The model under review builds one solid part; all positions refer to its coordinate system, in mm. Give positions to 0.01 mm unless a question says otherwise; leave off trailing zeros. Loops run counter-clockwise (first coordinate to the right, second up) from the corner with the lowest first, then second, coordinate; pieces in that order, holes last. Notation, with made-up numbers: (-29.5, 60.25) - (12.5, 60.25) arc R28 ccw to (12.5, 91.25) - close; hole circle Ø5 at (1, 12.25). An arc over 180 degrees is marked (long way). Return JSON: item names as keys, results as strings. Group by question number.
```python
from build123d import *

# Parameters (mm, degrees)
F0_W      = 72
F0_H      = 144
F1_DEPTH  = 6
F2_R      = 8
F3_R      = 5.8
F3_R_2    = 2
F4_DEPTH  = 25
F5_W      = 25
F5_H      = 3
F6_DEPTH  = 25
F7_W      = 8.5
F7_H      = 2.6
F8_DEPTH  = 25
F9_R      = 2
F9_W      = 10
F9_H      = 2.5
F10_DEPTH = 25
F12_DEPTH = 25
F14_DEPTH = 1.5
F16_DEPTH = 1
F17_SIZE  = 0.75


with BuildPart() as f1:
    # F0 (on Top) → F1 (new body)
    with BuildSketch(Plane.XY):
        Rectangle(F0_W, F0_H)
    extrude(amount=F1_DEPTH)

    # F2
    f2_edges = [f1.edges().sort_by_distance(p)[0] for p in [
        (-36, 72, 3),
        (36, 72, 3),
        (36, -72, 3),
        (-36, -72, 3),
    ]]
    fillet(f2_edges, radius=F2_R)

    # F3 (on Top) → F4 (cut)
    with BuildSketch(Plane.XY):
        with Locations((0, 47)):
            Circle(F3_R)
        with Locations((9.6, 47)):
            Circle(F3_R_2)
    extrude(amount=-F4_DEPTH, mode=Mode.SUBTRACT)

    # F5 (on face) → F6 (cut)
    with BuildSketch(Plane.YZ.offset(36)):
        with Locations((23.8, 2.5)):
            Rectangle(F5_W, F5_H)
    extrude(amount=-F6_DEPTH, mode=Mode.SUBTRACT)

    # F7 (on face) → F8 (cut)
    with BuildSketch(Plane.XZ.offset(72)):
        with Locations((15.25, 2.2)):
            Rectangle(F7_W, F7_H)
    extrude(amount=-F8_DEPTH, mode=Mode.SUBTRACT)

    # F9 (on face) → F10 (cut)
    with BuildSketch(Plane(origin=(0, 72, 0), x_dir=(-1, 0, 0), z_dir=(0, 1, 0))):
        with Locations((-14.83, 2.5)):
            Circle(F9_R)
        with Locations((21, 2.75)):
            Rectangle(F9_W, F9_H)
    extrude(amount=-F10_DEPTH, mode=Mode.SUBTRACT)

    # F11 (on face) → F12 (cut)
    with BuildSketch(Plane.XY.offset(6)):
        with BuildLine():
            Line((28, 70), (-28, 70))
            ThreePointArc((-28, 70), (-32.2426406871, 68.2426406871), (-34, 64))
            Line((-34, 64), (-34, -64))
            ThreePointArc((-34, -64), (-32.2426406871, -68.2426406871), (-28, -70))
            Line((-28, -70), (28, -70))
            ThreePointArc((28, -70), (32.2426406871, -68.2426406871), (34, -64))
            Line((34, -64), (34, 64))
            ThreePointArc((34, 64), (32.2426406871, 68.2426406871), (28, 70))
        make_face()
    extrude(amount=-F12_DEPTH, mode=Mode.SUBTRACT)

    # F13 (on face) → F14 (join)
    with BuildSketch(Plane.XY.offset(6)):
        with BuildLine():
            Line((28, 72), (-28, 72))
            ThreePointArc((-28, 72), (-33.6568542495, 69.6568542495), (-36, 64))
            Line((-36, 64), (-36, -64))
            ThreePointArc((-36, -64), (-33.6568542495, -69.6568542495), (-28, -72))
            Line((-28, -72), (28, -72))
            ThreePointArc((28, -72), (33.6568542495, -69.6568542495), (36, -64))
            Line((36, -64), (36, 64))
            ThreePointArc((36, 64), (33.6568542495, 69.6568542495), (28, 72))
        make_face()
        with BuildLine():
            ThreePointArc((-28, -68.5), (-31.1819805153, -67.1819805153), (-32.5, -64))
            Line((-32.5, -64), (-32.5, 64))
            ThreePointArc((-32.5, 64), (-31.1819805153, 67.1819805153), (-28, 68.5))
            Line((-28, 68.5), (28, 68.5))
            ThreePointArc((28, 68.5), (31.1819805153, 67.1819805153), (32.5, 64))
            Line((32.5, 64), (32.5, -64))
            ThreePointArc((32.5, -64), (31.1819805153, -67.1819805153), (28, -68.5))
            Line((28, -68.5), (-28, -68.5))
        make_face(mode=Mode.SUBTRACT)
    extrude(amount=F14_DEPTH)

    # F15 (on face) → F16 (join)
    with BuildSketch(Plane(origin=(0, 0, 0), x_dir=(1, 0, 0), z_dir=(0, 0, -1))):
        with BuildLine():
            Line((-28, -72), (28, -72))
            ThreePointArc((28, -72), (33.6568542495, -69.6568542495), (36, -64))
            Line((36, -64), (36, 64))
            ThreePointArc((36, 64), (33.6568542495, 69.6568542495), (28, 72))
            Line((28, 72), (-28, 72))
            ThreePointArc((-28, 72), (-33.6568542495, 69.6568542495), (-36, 64))
            Line((-36, 64), (-36, -64))
            ThreePointArc((-36, -64), (-33.6568542495, -69.6568542495), (-28, -72))
        make_face()
        with BuildLine():
            ThreePointArc((28, 70), (32.2426406871, 68.2426406871), (34, 64))
            Line((34, 64), (34, -64))
            ThreePointArc((34, -64), (32.2426406871, -68.2426406871), (28, -70))
            Line((28, -70), (-28, -70))
            ThreePointArc((-28, -70), (-32.2426406871, -68.2426406871), (-34, -64))
            Line((-34, -64), (-34, 64))
            ThreePointArc((-34, 64), (-32.2426406871, 68.2426406871), (-28, 70))
            Line((-28, 70), (28, 70))
        make_face(mode=Mode.SUBTRACT)
        with BuildLine():
            Line((34, -64), (34, 64))
            ThreePointArc((34, 64), (32.2426406871, 68.2426406871), (28, 70))
            Line((28, 70), (-28, 70))
            ThreePointArc((-28, 70), (-32.2426406871, 68.2426406871), (-34, 64))
            Line((-34, 64), (-34, -64))
            ThreePointArc((-34, -64), (-32.2426406871, -68.2426406871), (-28, -70))
            Line((-28, -70), (28, -70))
            ThreePointArc((28, -70), (32.2426406871, -68.2426406871), (34, -64))
        make_face()
        with BuildLine():
            ThreePointArc((-32, 64), (-30.8284271247, 66.8284271247), (-28, 68))
            Line((-28, 68), (28, 68))
            ThreePointArc((28, 68), (30.8284271247, 66.8284271247), (32, 64))
            Line((32, 64), (32, -64))
            ThreePointArc((32, -64), (30.8284271247, -66.8284271247), (28, -68))
            Line((28, -68), (-28, -68))
            ThreePointArc((-28, -68), (-30.8284271247, -66.8284271247), (-32, -64))
            Line((-32, -64), (-32, 64))
        make_face(mode=Mode.SUBTRACT)
    extrude(amount=F16_DEPTH)

    # F17
    f17_edges = [f1.edges().sort_by_distance(p)[0] for p in [
        (30.828427, -66.828427, 0),
        (31.181981, -67.181981, 6),
    ]]
    chamfer(f17_edges, length=F17_SIZE)


solid = f1.part
```
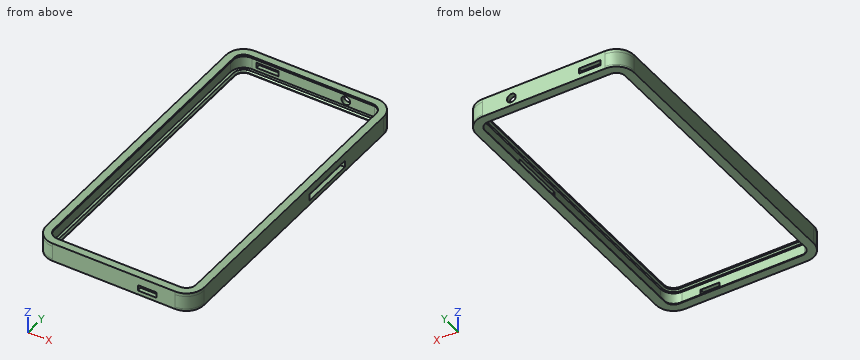
1) To check wall thickness, follow line 1 (X direction, y = -2, z = 7.25); line 2 (Y direction, x = 18.5, z = 5); line 3 (Y direction, x = -6.5, z = -0.25). State the ranges of each line that lie inside material, in increasing order.
2) For pin 1 Ø2 at (y, z) = (71, 3) entering from -X; pin 2 Ø1 at (y, z) = (19.5, 3) entering from +X; pin 3 Ø0.6 at (x, z) = (34.5, 2.5) entering from -Y, all flat-tipped, find the tip position at first contact; note any pin that passes through.
3) We need section A-A, the plane x = -2.5. Write out the cut boundary in (y, z), plus the area to 3 significant figures.
4) We need section C-C, the plane x = 14.83. Write out the cut boundary in (y, z).
5) We need section B-B, the plane y = 7. Write out the cut boundary in (x, z), plus the area to 3 significant figures.
6) We need section D-D, the plane x = -22.5. Write out the cut boundary in (y, z).
Findings:
{
 "1": {"line 1": "x = -36 to -32.5, 32.5 to 36", "line 2": "y = -72 to -70, 70 to 72", "line 3": "y = -72 to -68.5, 68.5 to 72"},
 "2": {"pin 1": "stops at x = -33.29", "pin 2": "stops at x = -34", "pin 3": "stops at y = -69.06"},
 "3": {"outline": "(-72, -1) - (-68, -1) - (-68, -0.75) - (-68.75, 0) - (-70, 0) - (-70, 6) - (-69.25, 6) - (-68.5, 6.75) - (-68.5, 7.5) - (-72, 7.5) - close; (68, -1) - (72, -1) - (72, 7.5) - (68.5, 7.5) - (68.5, 6.75) - (69.25, 6) - (70, 6) - (70, 0) - (68.75, 0) - (68, -0.75) - close", "area": "41.4 mm^2"},
 "4": {"outline": "(-72, -1) - (-68, -1) - (-68, -0.75) - (-68.75, 0) - (-70, 0) - (-70, 0.9) - (-72, 0.9) - close; (-72, 3.5) - (-70, 3.5) - (-70, 6) - (-69.25, 6) - (-68.5, 6.75) - (-68.5, 7.5) - (-72, 7.5) - close; (68, -1) - (72, -1) - (72, 0.5) - (70, 0.5) - (70, 0) - (68.75, 0) - (68, -0.75) - close; (68.5, 6.75) - (69.25, 6) - (70, 6) - (70, 4.5) - (72, 4.5) - (72, 7.5) - (68.5, 7.5) - close"},
 "5": {"outline": "(-36, -1) - (-32, -1) - (-32, -0.75) - (-32.75, 0) - (-34, 0) - (-34, 6) - (-33.25, 6) - (-32.5, 6.75) - (-32.5, 7.5) - (-36, 7.5) - close; (32, -1) - (36, -1) - (36, 7.5) - (32.5, 7.5) - (32.5, 6.75) - (33.25, 6) - (34, 6) - (34, 0) - (32.75, 0) - (32, -0.75) - close", "area": "41.4 mm^2"},
 "6": {"outline": "(-72, -1) - (-68, -1) - (-68, -0.75) - (-68.75, 0) - (-70, 0) - (-70, 6) - (-69.25, 6) - (-68.5, 6.75) - (-68.5, 7.5) - (-72, 7.5) - close; (68, -1) - (72, -1) - (72, 1.5) - (70, 1.5) - (70, 0) - (68.75, 0) - (68, -0.75) - close; (68.5, 6.75) - (69.25, 6) - (70, 6) - (70, 4) - (72, 4) - (72, 7.5) - (68.5, 7.5) - close"}
}
